```python
from build123d import *

# Parameters (mm, degrees)
SKETCH1_R           = 24
BOSS_EXTRUDE1_DEPTH = 54
SKETCH2_W           = 90.000197778
SKETCH2_H           = 36.253247866
CUT_EXTRUDE1_DEPTH  = 64.780874876
SKETCH3_R           = 3.5
SKETCH3_R_2         = 1
BOSS_EXTRUDE2_DEPTH = 14
CUT_EXTRUDE2_DEPTH  = 48
CUT_EXTRUDE3_START  = -3
SKETCH5_R           = 1
CUT_EXTRUDE3_DEPTH  = 3


with BuildPart() as part:
    # Sketch1 → Boss-Extrude1 (new body)
    with BuildSketch(Plane.XY):
        Circle(SKETCH1_R)
    extrude(amount=BOSS_EXTRUDE1_DEPTH)

    # Sketch2 → Cut-Extrude1 (cut, through all)
    with BuildSketch(Plane(origin=(0, 0, 0), x_dir=(-1, 0, 0), z_dir=(0, 0, -1))):
        with Locations((-2.008073343, 15.126623933)):
            Rectangle(SKETCH2_W, SKETCH2_H)
    extrude(amount=-CUT_EXTRUDE1_DEPTH, mode=Mode.SUBTRACT)

    # Sketch3 → Boss-Extrude2 (add)
    with BuildSketch(Plane(origin=(0, 0, 0), x_dir=(-1, 0, 0), z_dir=(0, 0, -1))):
        with Locations(Location((0, -12.5, 0), (0, 0, 180))):
            Circle(SKETCH3_R)
        with Locations((0, -12.5)):
            Circle(SKETCH3_R_2, mode=Mode.SUBTRACT)
    extrude(amount=BOSS_EXTRUDE2_DEPTH)

    # Sketch4 → Cut-Extrude2 (cut)
    with BuildSketch(Plane.XY.offset(51)):
        with BuildLine():
            Line((20.124611797, -6), (-20.124611797, -6))
            ThreePointArc((-20.124611797, -6), (0, -21), (20.124611797, -6))
        make_face()
    extrude(amount=-CUT_EXTRUDE2_DEPTH, mode=Mode.SUBTRACT)

    # Sketch5 → Cut-Extrude3 (cut)
    with BuildSketch(Plane(origin=(0, 0, 0), x_dir=(-1, 0, 0), z_dir=(0, 0, -1)).offset(CUT_EXTRUDE3_START)):
        with Locations((0, -12.5)):
            Circle(SKETCH5_R)
    extrude(amount=CUT_EXTRUDE3_DEPTH, mode=Mode.SUBTRACT)


solid = part.part
```
Geometry check sheet. Reference: the model listing, model coordinates, mm. A direction names the side the tool comes from. Coordinates: 2 decimals unless noted, no trailing zeros. Loops run counter-clockwise (first coordinate to the right, second up) from the corner with the lowest first, then second, coordinate; pieces in that order, holes last. Notation, with made-up numbers: (-8, -6) -> (-2, -6) arc R36 ccw to (-2, 31) -> close; hole circle Ø2 at (-4, -16). An arc over 180 degrees is marked (long way). Put each result on its own line as item: value.
1) Cross-section at A-A on x = 0. Record the boundary of the cut face in (y, z).
Result set:
outline: (-24, 0) -> (-16, 0) -> (-16, -14) -> (-13.5, -14) -> (-13.5, 3) -> (-21, 3) -> (-21, 51) -> (-6, 51) -> (-6, 3) -> (-11.5, 3) -> (-11.5, -14) -> (-9, -14) -> (-9, 0) -> (-3, 0) -> (-3, 54) -> (-24, 54) -> close
2) Thickness scan on line 1 (Z direction, x = -18, y = -8); line 2 (Y direction, x = 0, z = -6); line 3 (Z direction, x = 5, y = -23). Record the ranges inside material, lowest first.
Result set:
line 1: z = 0 to 3, 51 to 54
line 2: y = -16 to -13.5, -11.5 to -9
line 3: z = 0 to 54
3) Release check for a two-part mould opening along Y. For faces 1 (the cylindrical face through (0, -24, 27)), 2 (the flat face through (0, -12, 51)), 3 (the flat face through (-0.3, -8.7, 0)) record: released by +Y, released by -Y, zero draft, split by the parting line, or undercut.
Result set:
face 1: released by -Y
face 2: undercut
face 3: zero draft
4) Cross-section at C-C on z = -5. Record the boundary of the cut face in (x, y).
Result set:
outline: circle Ø7 at (0, -12.5); hole circle Ø2 at (0, -12.5)
5) Tool access check on faces 4 (the flat face through (0, -11, 54)), 5 (the cylindrical face through (-0.759, -9.083, -6.902)), 6 (the cylindrical face through (0, -21, 27)). Record the directions out of +Z, -Z, +X, -X, +Y, -Y that give a thin tool (end or side, any length) a straight path to the whole face; none if there is none.
Result set:
face 4: +Z, +X, -X, +Y, -Y
face 5: -Z
face 6: none
6) Gauge pin test, flat ends, axial feed: pin 1 Ø3 at (y, z) = (-15, -0.5) entering from +X; pin 2 Ø8 at (y, z) = (-21, 32) entering from +X; pin 3 Ø20 at (x, z) = (0.5, 30.5) entering from -Y. Record the tip position at first contact, or that the pin passes through.
Result set:
pin 1: stops at x = 19.78
pin 2: stops at x = 16.94
pin 3: stops at y = -24
7) Cross-section at D-D on x = -10.5. Record the boundary of the cut face in (y, z).
Result set:
outline: (-21.58, 0) -> (-3, 0) -> (-3, 54) -> (-21.58, 54) -> close; hole (-18.19, 3) -> (-6, 3) -> (-6, 51) -> (-18.19, 51) -> close
8) Cross-section at B-B on y = -9.75. Record the boundary of the cut face in (x, z), plus the area to 3 significant figures.
Result set:
outline: (-21.93, 0) -> (-2.17, 0) -> (-2.17, -14) -> (2.17, -14) -> (2.17, 0) -> (21.93, 0) -> (21.93, 54) -> (-21.93, 54) -> close; hole (-18.6, 3) -> (18.6, 3) -> (18.6, 51) -> (-18.6, 51) -> close
area: 644 mm^2
